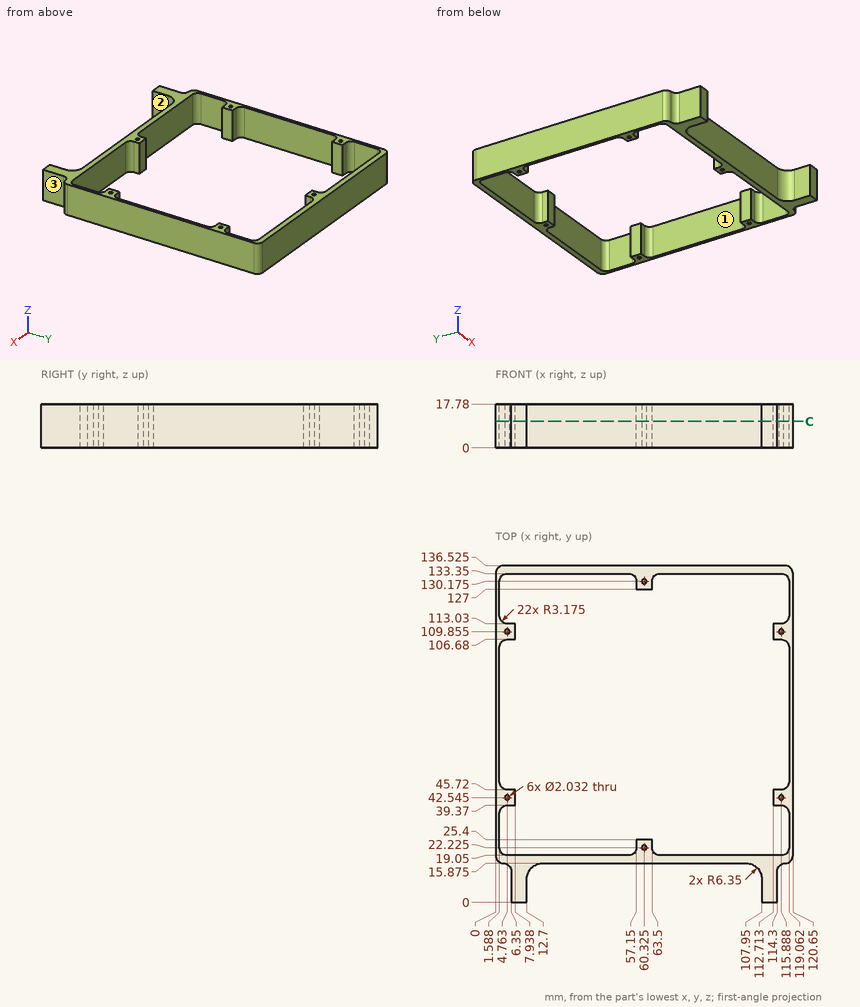
Design review of the part shown in the three views and the two pictorial views. Dimensions are in mm from the part's minimum x, y and z. A direction names the side the tool comes from. Coordinates: 2 decimals unless noted, no trailing zeros.
(1) Wall thickness on probe 1 along X at (y, z) = (23.5, 17); probe 2 along X at (y, z) = (29, 16.5); probe 3 along X at (y, z) = (10, 15): over which ranges is each line inside the solid? List them lowest first.
(2) Add section C-C on z = 10.75. Count the separate pieces of the cut face and the enclosed holes in it, then the cut area to 3 significant figures.
(3) For pin 1 Ø5.5 at (x, z) = (70.5, 11) entering from -Y (1 decimal); pin 2 Ø1.6 at (x, y) = (4.76, 109.86) entering from -Z; pin 3 Ø3 at (y, z) = (6.5, 11) entering from -X; pin 4 Ø5 at (y, z) = (14.5, 13.5) entering from -X, all flat-tipped, find the tip position at first contact; note any pin that passes through.
(4) Tool access review of the marked faces 1, 2 and 3: name each direction out of +Z, -Z, +X, -X, +Y, -Y from which nothing blocks a thin tool from reaching the whole face with its end or side.
Answer sheet:
1. probe 1: x = 0 to 1.59, 57.15 to 63.5, 119.06 to 120.65
1. probe 2: x = 0 to 1.59, 119.06 to 120.65
1. probe 3: x = 6.35 to 12.72, 107.93 to 114.3
2. separate pieces: 1
2. enclosed holes: 7
2. area: 1,600 mm2
3. pin 1: stops at y = 15.9
3. pin 2: passes through
3. pin 3: stops at x = 6.35
3. pin 4: stops at x = 0.75
4. face 1: +Z, -Z
4. face 2: +Z, -Z, -Y
4. face 3: +Z, -Z, +X, -Y
